from build123d import *

# Parameters (mm, degrees)
SKETCH1_W           = 5
SKETCH1_H           = 5
BOSS_EXTRUDE1_DEPTH = 110
SKETCH2_W           = 3
SKETCH2_H           = 3
CUT_EXTRUDE1_DEPTH  = 9
SKETCH3_W           = 3
SKETCH3_H           = 3
CUT_EXTRUDE2_DEPTH  = 9
SKETCH4_W           = 5
SKETCH4_H           = 5
BOSS_EXTRUDE2_DEPTH = 6
SKETCH5_R           = 1.4
BOSS_EXTRUDE3_DEPTH = 13


with BuildPart() as part:
    # Sketch1 → Boss-Extrude1 (new body)
    with BuildSketch(Plane.XY):
        with Locations((2.5, 2.5)):
            Rectangle(SKETCH1_W, SKETCH1_H)
    extrude(amount=BOSS_EXTRUDE1_DEPTH)

    # Sketch2 → Cut-Extrude1 (cut)
    with BuildSketch(Plane.ZY):
        with Locations((2.5, 2.5)):
            Rectangle(SKETCH2_W, SKETCH2_H)
        with Locations((107.5, 2.5)):
            Rectangle(SKETCH2_W, SKETCH2_H)
        with Locations((13.5, 2.5)):
            Rectangle(SKETCH2_W, SKETCH2_H)
        with Locations((96.5, 2.5)):
            Rectangle(SKETCH2_W, SKETCH2_H)
    extrude(amount=-CUT_EXTRUDE1_DEPTH, mode=Mode.SUBTRACT)

    # Sketch3 → Cut-Extrude2 (cut)
    with BuildSketch(Plane(origin=(0, 5, 0), x_dir=(1, 0, 0), z_dir=(0, 1, 0))):
        with Locations((2.5, -25.15)):
            Rectangle(SKETCH3_W, SKETCH3_H)
        with Locations((2.5, -55)):
            Rectangle(SKETCH3_W, SKETCH3_H)
    extrude(amount=-CUT_EXTRUDE2_DEPTH, mode=Mode.SUBTRACT)

    # Sketch4 → Boss-Extrude2 (add)
    with BuildSketch(Plane(origin=(0, 0, 0), x_dir=(-1, 0, 0), z_dir=(0, -1, 0))):
        with Locations((-2.5, -70.15)):
            Rectangle(SKETCH4_W, SKETCH4_H)
    extrude(amount=BOSS_EXTRUDE2_DEPTH)

    # Sketch5 → Boss-Extrude3 (add)
    with BuildSketch(Plane.ZY):
        with Locations((70.15, -3)):
            Circle(SKETCH5_R)
    extrude(amount=-BOSS_EXTRUDE3_DEPTH)


solid = part.part
Work out the finished part from the listing and answer in its coordinate system (mm). A direction names the side the tool comes from. Give positions to 0.01 mm unless a question says otherwise; leave off trailing zeros. Order: outer loops, then holes, each group sorted by start corner. A loop starts at its lowest first (then second) coordinate and runs counter-clockwise, first axis right, second up. Notation, with made-up numbers: (82, -8.75) -> (125, -8.75) arc R14 cw to (125, 14.25) -> close; hole circle Ø2 at (61.25, 67.5). An arc over 180 degrees is marked (long way). One line per item, written item: value.
Item 1: Straight lines are drawn through the part: probe 1 along X at (y, z) = (0.5, 33); probe 2 along Z at (x, y) = (2, -1.75). For each, find the intervals that lie inside material, in ascending order.
Answer sheet:
probe 1: 0 to 5
probe 2: 67.65 to 72.65
Item 2: Find section B-B, the plane y = -3. Give the vertices of the cut face in (x, z).
Answer sheet:
outline: (0, 67.65) -> (5, 67.65) -> (5, 68.75) -> (13, 68.75) -> (13, 71.55) -> (5, 71.55) -> (5, 72.65) -> (0, 72.65) -> close
Item 3: Find section C-C, the plane z = 70.15. Give the vertices of the cut face in (x, y), plus the area to 3 significant figures.
Answer sheet:
outline: (0, -6) -> (5, -6) -> (5, -4.4) -> (13, -4.4) -> (13, -1.6) -> (5, -1.6) -> (5, 5) -> (0, 5) -> close
area: 77.4 mm²
Item 4: Determine the mould class of faces 1 (the flat face through (2, 2, 15)), 2 (the flat face through (3, -3, 67.65)), 3 (the flat face through (0.8, 5, 54.2)) for opening direction Z: released by +Z, released by -Z, zero draft, split by the parting line, or undercut.
Answer sheet:
face 1: undercut
face 2: released by -Z
face 3: zero draft
Item 5: Find section D-D, the plane x = 8.5. Give the vertices of the cut face in (y, z), plus the area to 3 significant figures.
Answer sheet:
outline: circle Ø2.8 at (-3, 70.15)
area: 6.16 mm²
Item 6: Flat-ended cylindrical pins translate along their axes: P1, Ø2.5, axis at x = 2, y = 2, coming from the -Z side; P2, Ø2.5, axis at x = 3, z = 2.5, coming from the -Y side; P3, Ø1.5, axis at y = 2.5, z = 26, coming from the +X side; P4, Ø1, axis at x = 11, z = 69.5, coming from the -Y side. Find the tip coordinate at first contact, or state that the pin passes through.
Answer sheet:
P1: z = 0
P2: y = 0
P3: x = 5
P4: y = -4.39
Item 7: Find section A-A, the plane x = 2.25. State how many separate pieces and enclosed holes the cut face has, plus the area to 3 significant figures.
Answer sheet:
separate pieces: 3
enclosed holes: 4
area: 514 mm²
Item 8: A tool of negligible diameter and unlimited length cuts with its end or side. For faces 4 (the flat face through (2, 0, 33)), 5 (the flat face through (2, 0, 91)), 6 (the flat face through (2, 1, 107)), 7 (the flat face through (2, 3, 26.65)), from which of +Z, -Z, +X, -X, +Y, -Y can it reach the whole face along a straight path? Write none if from no direction.
Answer sheet:
face 4: -Z, +X, -X, -Y
face 5: +Z, +X, -X, -Y
face 6: +X, -X
face 7: +Y, -Y
